Read the model definition and answer for the solid it produces. Units are mm, in the model's axes. A direction names the side the tool comes from. Coordinates: 2 decimals unless noted, no trailing zeros. Order: outer loops, then holes, each group sorted by start corner. A loop starts at its lowest first (then second) coordinate and runs counter-clockwise, first axis right, second up. Notation, with made-up numbers: M 22.5,28.25 L 76.5,28.25 A24 ccw 76.5,56.25 Z; hole C -31,-19.75 d1. An arc over 180 degrees is marked long. Put each result on its own line as item: value.
from build123d import *

# Parameters (mm, degrees)
EXTRUDE_1_DEPTH     = 20
FILLET_1_R          = 10
FILLET_2_R          = 0.5
CUT_EXTRUDE_1_DEPTH = 5
CUT_EXTRUDE_2_DEPTH = 5
CUT_EXTRUDE_3_DEPTH = 46.044422689
CHAMFER_1_SIZE      = 5
CHAMFER_2_SIZE      = 2


with BuildPart() as part:
    # Sketch 1 → Extrude 1 (new body)
    with BuildSketch(Plane(origin=(0, 0, 0), x_dir=(0, 0, -1), z_dir=(1, 0, 0))):
        with BuildLine():
            ThreePointArc((-8.892304845, -8.598076211), (-12.990381057, -7.5), (-11.892304845, -3.401923789))
            Line((-11.892304845, -3.401923789), (-1.5, 2.598076211))
            ThreePointArc((-1.5, 2.598076211), (0.776457135, 2.897777479), (2.598076211, 1.5))
            Line((2.598076211, 1.5), (14, 1.5))
            Line((14, 1.5), (14, 5))
            Line((14, 5), (9, 10))
            Line((9, 10), (-30, 10))
            Line((-30, 10), (-30, -17))
            Line((-30, -17), (14, -17))
            Line((14, -17), (14, -1.5))
            Line((14, -1.5), (2.598076211, -1.5))
            ThreePointArc((2.598076211, -1.5), (2.121320344, -2.121320344), (1.5, -2.598076211))
            Line((1.5, -2.598076211), (-3.62758528, -5.558488953))
            Line((-3.62758528, -5.558488953), (-8.892304845, -8.598076211))
        make_face()
        with BuildLine():
            Line((-3, 0), (-3.62758528, -5.558488953))
            Line((-3.62758528, -5.558488953), (1.5, -2.598076211))
            ThreePointArc((1.5, -2.598076211), (-1.5, -2.598076211), (-3, 0))
        make_face()
    extrude(amount=EXTRUDE_1_DEPTH)

    # Fillet 1
    fillet_1_edges = [part.edges().sort_by_distance(p)[0] for p in [
        (10, -5.558488953, 3.62758528),
    ]]
    fillet(fillet_1_edges, radius=FILLET_1_R)

    # Fillet 2
    fillet_2_edges = [part.edges().sort_by_distance(p)[0] for p in [
        (10, 0, 3),
    ]]
    fillet(fillet_2_edges, radius=FILLET_2_R)

    # Sketch 2 → Cut-Extrude 1 (cut)
    with BuildSketch(Plane(origin=(0, 10, 0), x_dir=(1, 0, 0), z_dir=(0, 1, 0))):
        with BuildLine():
            ThreePointArc((14.35, -11), (13.075914498, -7.924085502), (10, -6.65))
            Line((10, -6.65), (10, -8.5))
            ThreePointArc((10, -8.5), (11.767766953, -9.232233047), (12.5, -11))
            ThreePointArc((12.5, -11), (11.767766953, -12.767766953), (10, -13.5))
            Line((10, -13.5), (10, -15.35))
            ThreePointArc((10, -15.35), (13.075914498, -14.075914498), (14.35, -11))
        make_face()
        with BuildLine():
            Line((10, -8.5), (10, -6.65))
            ThreePointArc((10, -6.65), (5.65, -11), (10, -15.35))
            Line((10, -15.35), (10, -13.5))
            ThreePointArc((10, -13.5), (7.5, -11), (10, -8.5))
        make_face()
        with BuildLine():
            ThreePointArc((14.35, -23), (13.075914498, -19.924085502), (10, -18.65))
            Line((10, -18.65), (10, -20.5))
            ThreePointArc((10, -20.5), (11.767766953, -21.232233047), (12.5, -23))
            ThreePointArc((12.5, -23), (11.767766953, -24.767766953), (10, -25.5))
            Line((10, -25.5), (10, -27.35))
            ThreePointArc((10, -27.35), (13.075914498, -26.075914498), (14.35, -23))
        make_face()
        with BuildLine():
            Line((10, -20.5), (10, -18.65))
            ThreePointArc((10, -18.65), (5.65, -23), (10, -27.35))
            Line((10, -27.35), (10, -25.5))
            ThreePointArc((10, -25.5), (7.5, -23), (10, -20.5))
        make_face()
    extrude(amount=-CUT_EXTRUDE_1_DEPTH, mode=Mode.SUBTRACT)

    # Sketch 2_3 → Cut-Extrude 2 (cut)
    with BuildSketch(Plane(origin=(0, 10, 0), x_dir=(1, 0, 0), z_dir=(0, 1, 0))):
        with BuildLine():
            ThreePointArc((17.668801229, 9), (15, 10.85), (12.331198771, 9))
            Line((12.331198771, 9), (13.881966011, 9))
            ThreePointArc((13.881966011, 9), (15, 9.5), (16.118033989, 9))
            Line((16.118033989, 9), (17.668801229, 9))
        make_face()
        with BuildLine():
            Line((13.881966011, 9), (12.331198771, 9))
            ThreePointArc((12.331198771, 9), (14.491858043, 5.195665542), (17.85, 8))
            ThreePointArc((17.85, 8), (17.804334458, 8.508141957), (17.668801229, 9))
            Line((17.668801229, 9), (16.118033989, 9))
            ThreePointArc((16.118033989, 9), (16.401258538, 8.535233135), (16.5, 8))
            ThreePointArc((16.5, 8), (14.464766865, 6.598741462), (13.881966011, 9))
        make_face()
        with BuildLine():
            ThreePointArc((6.118033989, 9), (6.401258538, 8.535233135), (6.5, 8))
            ThreePointArc((6.5, 8), (4.464766865, 6.598741462), (3.881966011, 9))
            Line((3.881966011, 9), (2.331198771, 9))
            ThreePointArc((2.331198771, 9), (4.491858043, 5.195665542), (7.85, 8))
            ThreePointArc((7.85, 8), (7.804334458, 8.508141957), (7.668801229, 9))
            Line((7.668801229, 9), (6.118033989, 9))
        make_face()
        with BuildLine():
            ThreePointArc((3.881966011, 9), (5, 9.5), (6.118033989, 9))
            Line((6.118033989, 9), (7.668801229, 9))
            ThreePointArc((7.668801229, 9), (5, 10.85), (2.331198771, 9))
            Line((2.331198771, 9), (3.881966011, 9))
        make_face()
    extrude(amount=-CUT_EXTRUDE_2_DEPTH, mode=Mode.SUBTRACT)

    # Sketch 2_4 → Cut-Extrude 3 (cut, through all)
    with BuildSketch(Plane(origin=(0, 10, 0), x_dir=(1, 0, 0), z_dir=(0, 1, 0))):
        with BuildLine():
            Line((16.118033989, 9), (13.881966011, 9))
            ThreePointArc((13.881966011, 9), (14.464766865, 6.598741462), (16.5, 8))
            ThreePointArc((16.5, 8), (16.401258538, 8.535233135), (16.118033989, 9))
        make_face()
        with BuildLine():
            ThreePointArc((16.118033989, 9), (15, 9.5), (13.881966011, 9))
            Line((13.881966011, 9), (16.118033989, 9))
        make_face()
        with BuildLine():
            Line((3.881966011, 9), (6.118033989, 9))
            ThreePointArc((6.118033989, 9), (5, 9.5), (3.881966011, 9))
        make_face()
        with BuildLine():
            ThreePointArc((6.5, 8), (6.401258538, 8.535233135), (6.118033989, 9))
            Line((6.118033989, 9), (3.881966011, 9))
            ThreePointArc((3.881966011, 9), (4.464766865, 6.598741462), (6.5, 8))
        make_face()
        with BuildLine():
            ThreePointArc((12.5, -11), (11.767766953, -9.232233047), (10, -8.5))
            Line((10, -8.5), (10, -13.5))
            ThreePointArc((10, -13.5), (11.767766953, -12.767766953), (12.5, -11))
        make_face()
        with BuildLine():
            Line((10, -13.5), (10, -8.5))
            ThreePointArc((10, -8.5), (7.5, -11), (10, -13.5))
        make_face()
        with BuildLine():
            ThreePointArc((12.5, -23), (11.767766953, -21.232233047), (10, -20.5))
            Line((10, -20.5), (10, -25.5))
            ThreePointArc((10, -25.5), (11.767766953, -24.767766953), (12.5, -23))
        make_face()
        with BuildLine():
            Line((10, -25.5), (10, -20.5))
            ThreePointArc((10, -20.5), (7.5, -23), (10, -25.5))
        make_face()
    extrude(amount=-CUT_EXTRUDE_3_DEPTH, mode=Mode.SUBTRACT)

    # Chamfer 1
    chamfer_1_edges = [part.edges().sort_by_distance(p)[0] for p in [
        (0, -3.5, 30),
        (20, -3.5, 30),
    ]]
    chamfer(chamfer_1_edges, length=CHAMFER_1_SIZE)

    # Chamfer 2
    chamfer_2_edges = [part.edges().sort_by_distance(p)[0] for p in [
        (0, -9.25, -14),
        (0, 3.25, -14),
        (20, 3.25, -14),
        (20, -9.25, -14),
    ]]
    chamfer(chamfer_2_edges, length=CHAMFER_2_SIZE)


solid = part.part
Q1. For a pull along Z with two mould halves and no side action, classify faces 6 (the face through (10, -9, -14)), 7 (the face through (10, -1.5, -8)), 8 (the face through (12, 5, 25)) as +Z half, -Z half, draft (parallel to the pull), parting line (faces both ways), or undercut.
Answers below:
face 6: -Z half
face 7: draft
face 8: undercut
Q2. Given pin 1 (2.5 mm diameter, centred on x = 8, z = 23, fed in from +Y); pin 2 (1.8 mm diameter, centred on x = 5, z = -8, fed in from +Y), each flat-ended and moving along its own axis, determine where each tip first touches the part or whether it passes through.
Answers below:
pin 1: stops at y = 5
pin 2: passes through
Q3. Consider line 1 along X through (y, z) = (7.6, -8); line 2 along X through (y, z) = (7, -7); line 3 along Z through (x, y) = (5, -10.25). Determine where each line is inside the solid, lowest interval first.
Answers below:
line 1: x = 0 to 2.15, 7.85 to 12.15, 17.85 to 20
line 2: x = 0 to 2.33, 7.67 to 12.33, 17.67 to 20
line 3: z = -14 to -9.5, -6.5 to 30
Q4. Find section C-C on y = -11.5. Write down the section's boundary in (x, z), plus the area to 3 significant figures.
Answers below:
outline: M 0,-12 L 2,-14 L 18,-14 L 20,-12 L 20,25 L 15,30 L 5,30 L 0,25 Z; hole C 5,-8 d3; hole C 10,11 d5; hole C 10,23 d5; hole C 15,-8 d3
area: 798 mm^2
Q5. Find section D-D on y = -0.25. Write down the section's boundary in (x, z).
Answers below:
outline: M 0,6.43 L 20,6.43 L 20,25 L 15,30 L 5,30 L 0,25 Z; hole C 10,11 d5; hole C 10,23 d5
Q6. A tool of negligible diameter and unlimited length cuts with its end or side. For faces 1 (the face through (3, -3, 28)), 2 (the face through (18, -3, 27)), 3 (the face through (9.86, -8.28, 8.34)), 4 (the face through (10, 1.5, -8)), 5 (the face through (16.2, 5, -6.8)), from which of +Z, -Z, +X, -X, +Y, -Y can it reach the whole face along a straight path? Write none if from no direction.
Answers below:
face 1: +Z, -X, +Y, -Y
face 2: +Z, +X, +Y, -Y
face 3: +X, -X
face 4: -Z, +X, -X
face 5: +Y
Q7. Find section B-B on z = 22. Write down the section's boundary in (x, y).
Answers below:
outline: M 0,-17 L 7.71,-17 L 7.71,5 L 5.77,5 L 5.77,10 L 0,10 Z; M 12.29,-17 L 20,-17 L 20,10 L 14.23,10 L 14.23,5 L 12.29,5 Z
Q8. Find section A-A on y = -6. Write down the section's boundary in (x, z).
Answers below:
outline: M 0,-12 L 2,-14 L 18,-14 L 20,-12 L 20,5.47 L 0,5.47 Z; M 0,13.39 L 9.27,13.39 A2.5 cw 10.73,13.39 L 20,13.39 L 20,25 L 15,30 L 5,30 L 0,25 Z; hole C 5,-8 d3; hole C 10,23 d5; hole C 15,-8 d3
